Verification items for the finished model (mm, model axes). A direction names the side the tool comes from. Coordinates: 2 decimals unless noted, no trailing zeros. Order: outer loops, then holes, each group sorted by start corner. A loop starts at its lowest first (then second) coordinate and runs counter-clockwise, first axis right, second up. Notation, with made-up numbers: M 77.25,-34 L 115.25,-34 A25 cw 115.25,-6 Z; hole C 31,55 d10. An arc over 180 degrees is marked long. Return JSON: item names as keys, results as strings. Group by question number.
1. Gauge pin test, flat ends, axial feed: pin 1 (13 mm diameter, centred on x = -17, z = 17.5, fed in from -Y); pin 2 (1.2 mm diameter, centred on x = 0, z = 9.5, fed in from -Y); pin 3 (0.8 mm diameter, centred on x = -28.5, y = 2, fed in from +Z). Record the tip position at first contact, or that the pin passes through.
2. Section check A-A, the plane y = 2. Record the cut outline in (x, z).
3. Mould release check, pull along Z, two halves, no side actions. Record for faces 4 (the flat face through (-11, 4, 28.069)), 5 (the flat face through (-29.237, 5, 11)), 6 (the flat face through (-27.737, 4.7, 11)): +Z half, -Z half, draft (parallel to the pull), parting line (faces both ways), or undercut.
4. Section check D-D, the plane y = 6.5. Record the cut outline in (x, z), plus the area to 3 significant figures.
5. Section check B-B, the plane z = 11. Record the cut outline in (x, y).
6. Section check C-C, the plane x = -17.75. Record the cut outline in (y, z).
7. Material ranges on line 1 along X through (y, z) = (2.25, 2.25); line 2 along Z through (x, y) = (-13, 3.5); line 3 along Z through (x, y) = (-0.5, 1.75), recorded low to high.
8. Set-up check for faces 1 (the flat face through (-0.737, 2, 17)), 2 (the flat face through (0.763, 5, 14)), 3 (the flat face through (0, 2, 6.569)): record each of +Z, -Z, +X, -X, +Y, -Y from which the full face is reachable in a straight line by a thin tool's end or side.
```python
from build123d import *

# Parameters (mm, degrees)
SKETCH1_W           = 30
SKETCH1_H           = 29
BOSS_EXTRUDE1_DEPTH = 8
SKETCH2_W           = 24
SKETCH2_H           = 8
CUT_EXTRUDE1_DEPTH  = 8
CUT_EXTRUDE2_DEPTH  = 8
CUT_EXTRUDE3_DEPTH  = 5
SKETCH5_W           = 9
SKETCH5_H           = 4
CUT_EXTRUDE4_DEPTH  = 30
SKETCH2_2_W         = 24
SKETCH2_2_H         = 8
BOSS_EXTRUDE2_DEPTH = 3


with BuildPart() as part:
    # Sketch1 → Boss-Extrude1 (new body)
    with BuildSketch(Plane(origin=(0, 0, 0), x_dir=(1, 0, 0), z_dir=(0, 1, 0))):
        with Locations((-14.236607143, -13.569196429)):
            Rectangle(SKETCH1_W, SKETCH1_H)
    extrude(amount=BOSS_EXTRUDE1_DEPTH)

    # Sketch2 → Cut-Extrude1 (cut)
    with BuildSketch(Plane(origin=(0, 8, 0), x_dir=(1, 0, 0), z_dir=(0, 1, 0))):
        with Locations((-14.236607143, -6.069196429)):
            Rectangle(SKETCH2_W, SKETCH2_H)
        with Locations((-14.236607143, -17.069196429)):
            Rectangle(SKETCH2_W, SKETCH2_H)
    extrude(amount=-CUT_EXTRUDE1_DEPTH, mode=Mode.SUBTRACT)

    # Sketch3 → Cut-Extrude2 (cut)
    with BuildSketch(Plane(origin=(0, 8, 0), x_dir=(1, 0, 0), z_dir=(0, 1, 0))):
        Polygon((-29.236607143, -22.519140749), (-22.236607143, -28.069196429), (-29.236607143, -28.069196429), align=None)
    extrude(amount=-CUT_EXTRUDE2_DEPTH, mode=Mode.SUBTRACT)

    # Sketch4 → Cut-Extrude3 (cut)
    with BuildSketch(Plane.XZ):
        Polygon((-0.736607143, 0.569196429), (-27.736607143, 0.569196429), (-27.736607143, 21.794168589), (-21.714109927, 26.569196429), (-0.736607143, 26.569196429), align=None)
    extrude(amount=-CUT_EXTRUDE3_DEPTH, mode=Mode.SUBTRACT)

    # Sketch5 → Cut-Extrude4 (cut)
    with BuildSketch(Plane.ZY.offset(29.236607143)):
        with Locations((11.069196429, 2)):
            Rectangle(SKETCH5_W, SKETCH5_H)
    extrude(amount=-CUT_EXTRUDE4_DEPTH, mode=Mode.SUBTRACT)

    # Sketch2<2> → Boss-Extrude2 (add)
    with BuildSketch(Plane(origin=(0, 8, 0), x_dir=(1, 0, 0), z_dir=(0, 1, 0))):
        with Locations((-14.236607143, -6.069196429)):
            Rectangle(SKETCH2_2_W, SKETCH2_2_H)
        with Locations((-14.236607143, -17.069196429)):
            Rectangle(SKETCH2_2_W, SKETCH2_2_H)
    extrude(amount=-BOSS_EXTRUDE2_DEPTH)


solid = part.part
```
Answers follow:
{
 "1": {"pin 1": "y = 5", "pin 2": "y = 4", "pin 3": "z = 23.42"},
 "2": {"outline": "M -29.24,-0.93 L 0.76,-0.93 L 0.76,6.57 L -0.74,6.57 L -0.74,0.57 L -27.74,0.57 L -27.74,6.57 L -29.24,6.57 Z; M -29.24,15.57 L -27.74,15.57 L -27.74,21.79 L -21.71,26.57 L -0.74,26.57 L -0.74,15.57 L 0.76,15.57 L 0.76,28.07 L -22.24,28.07 L -29.24,22.52 Z"},
 "3": {"face 4": "+Z half", "face 5": "draft", "face 6": "undercut"},
 "4": {"outline": "M -29.24,-0.93 L 0.76,-0.93 L 0.76,28.07 L -22.24,28.07 L -29.24,22.52 Z", "area": "851 mm^2"},
 "5": {"outline": "M -29.24,4 L -27.74,4 L -27.74,5 L -0.74,5 L -0.74,4 L 0.76,4 L 0.76,8 L -29.24,8 Z"},
 "6": {"outline": "M 0,-0.93 L 8,-0.93 L 8,28.07 L 0,28.07 L 0,26.57 L 5,26.57 L 5,0.57 L 0,0.57 Z"},
 "7": {"line 1": "-29.24 to -27.74, -0.74 to 0.76", "line 2": "-0.93 to 0.57, 26.57 to 28.07", "line 3": "-0.93 to 6.57, 15.57 to 28.07"},
 "8": {"face 1": "-Y", "face 2": "+Z, -Z, +X, +Y, -Y", "face 3": "+X, -X, -Y"}
}
